```python
from build123d import *

# Parameters (mm, degrees)
SKETCH1_R           = 3.75
SKETCH1_R_2         = 1.6
BOSS_EXTRUDE1_DEPTH = 2
BOSS_EXTRUDE2_START = -15
BOSS_EXTRUDE2_DEPTH = 15
BOSS_EXTRUDE3_DEPTH = 2
SKETCH2_R           = 2
CUT_EXTRUDE1_DEPTH  = 39.169212171
CUT_EXTRUDE2_START  = -4
SKETCH2_3_R         = 2
CUT_EXTRUDE2_DEPTH  = 35.169212171


# Read off the part's stored shape, not the designer's step: Boss-Extrude2
with BuildPart() as part:
    # Sketch1 → Boss-Extrude1 (new body)
    # profile 1 of 5: a face of its own
    with BuildSketch(Plane.XY):
        with Locations((-33.25, 6.273123532)):
            Circle(SKETCH1_R)
        with Locations((-33.25, 6.273123532)):
            Circle(SKETCH1_R_2, mode=Mode.SUBTRACT)
    # profile 2 of 5: a face of its own
    with BuildSketch(Plane.XY):
        with BuildLine():
            Line((0, 2.523123532), (3.75, 2.523123532))
            ThreePointArc((3.75, 2.523123532), (0.004577287, 6.087897443), (3.38, 10.004825556))
            Line((3.38, 10.004825556), (0, 10.023123532))
            Line((0, 10.023123532), (0, 13))
            Line((0, 13), (-29.5, 13))
            Line((-29.5, 13), (-29.5, 10.023123532))
            Line((-29.5, 10.023123532), (-33.25, 10.023123532))
            ThreePointArc((-33.25, 10.023123532), (-30.598349571, 8.924773961), (-29.5, 6.273123532))
            ThreePointArc((-29.5, 6.273123532), (-30.598349571, 3.621473102), (-33.25, 2.523123532))
            Line((-33.25, 2.523123532), (-29.5, 2.523123532))
            Line((-29.5, 2.523123532), (-29.5, 0))
            Line((-29.5, 0), (0, 0))
            Line((0, 0), (0, 2.523123532))
        make_face()
    # profile 3 of 5: a face of its own
    with BuildSketch(Plane.XY):
        with Locations((3.75, 6.273123532)):
            Circle(SKETCH1_R)
        with Locations((3.75, 6.273123532)):
            Circle(SKETCH1_R_2, mode=Mode.SUBTRACT)
    # profile 4 of 5: a face of its own
    with BuildSketch(Plane.XY):
        with BuildLine():
            ThreePointArc((7.5, 6.273123532), (6.401650429, 3.621473102), (3.75, 2.523123532))
            Line((3.75, 2.523123532), (0, 2.523123532))
            Line((0, 2.523123532), (0, 0))
            Line((0, 0), (7.5, 0))
            Line((7.5, 0), (7.5, 6.273123532))
        make_face()
    # profile 5 of 5: a face of its own
    with BuildSketch(Plane.XY):
        with BuildLine():
            Line((-37, 0), (-29.5, 0))
            Line((-29.5, 0), (-29.5, 2.523123532))
            Line((-29.5, 2.523123532), (-33.25, 2.523123532))
            ThreePointArc((-33.25, 2.523123532), (-35.901650429, 3.621473102), (-37, 6.273123532))
            Line((-37, 6.273123532), (-37, 0))
        make_face()
    extrude(amount=BOSS_EXTRUDE1_DEPTH)



with BuildPart() as body_2:
    # Boss-Extrude2 outline → Boss-Extrude2 (new body)
    with BuildSketch(Plane(origin=(0, 0, 0), x_dir=(1, 0, 0), z_dir=(0, 1, 0)).offset(BOSS_EXTRUDE2_START)):
        Polygon((7.5, 0), (7.5, 26.552667029), (-37, 5.801976241), (-37, 0), align=None)
    extrude(amount=BOSS_EXTRUDE2_DEPTH)


with BuildPart() as part_1:
    add(part.part)

    add(body_2.part)  # Boss-Extrude3 merges body 2
    # Sketch1<5> → Boss-Extrude3 (add)
    with BuildSketch(Plane.XY):
        Polygon((7.5, 0), (0, 0), (-29.5, 0), (-37, 0), (-37, -15), (7.5, -15), align=None)
    extrude(amount=BOSS_EXTRUDE3_DEPTH)

    # Sketch2 → Cut-Extrude1 (cut, through all)
    with BuildSketch(Plane(origin=(-8.83071505, 0, -18.937529538), x_dir=(-0.9063077870366508, 0, 0.42261826174069766), z_dir=(-0.4226182617406977, 1.198406961524809e-15, -0.9063077870366509))):
        with Locations((16.531049613, -7.5)):
            Circle(SKETCH2_R)
        with Locations((-3.468950387, -7.5)):
            Circle(SKETCH2_R)
    extrude(amount=-CUT_EXTRUDE1_DEPTH, mode=Mode.SUBTRACT)

    # Sketch2<3> → Cut-Extrude2 (cut, through all)
    # profile 1 of 2: a face of its own
    with BuildSketch(Plane(origin=(-8.83071505, 0, -18.937529538), x_dir=(-0.9063077870366508, 0, 0.42261826174069766), z_dir=(-0.4226182617406977, 1.198406961524809e-15, -0.9063077870366509)).offset(CUT_EXTRUDE2_START)):
        Polygon((12.605067782, -7.5), (14.568058697, -10.9), (18.494040528, -10.9), (20.457031443, -7.5), (18.494040528, -4.1), (14.568058697, -4.1), align=None)
        with Locations((16.531049613, -7.5)):
            Circle(SKETCH2_3_R, mode=Mode.SUBTRACT)
    # profile 2 of 2: a face of its own
    with BuildSketch(Plane(origin=(-8.83071505, 0, -18.937529538), x_dir=(-0.9063077870366508, 0, 0.42261826174069766), z_dir=(-0.4226182617406977, 1.198406961524809e-15, -0.9063077870366509)).offset(CUT_EXTRUDE2_START)):
        Polygon((-5.431941303, -4.1), (-7.394932218, -7.5), (-5.431941303, -10.9), (-1.505959472, -10.9), (0.457031443, -7.5), (-1.505959472, -4.1), align=None)
        with Locations((-3.468950387, -7.5)):
            Circle(SKETCH2_3_R, mode=Mode.SUBTRACT)
    extrude(amount=-CUT_EXTRUDE2_DEPTH, mode=Mode.SUBTRACT)


solid = part_1.part
```
Geometry: final body of the model. Coordinates: model frame, mm. A direction names the side the tool comes from. Round coordinates to 2 decimals unless told otherwise and drop trailing zeros. Order: outer loops, then holes, each group sorted by start corner. A loop starts at its lowest first (then second) coordinate and runs counter-clockwise, first axis right, second up. Notation, with made-up numbers: M 44,36 L 92,36 A37 ccw 92,73 Z; hole C 32,21.5 d1. An arc over 180 degrees is marked long. Use one line per item in the form item = value. Start each with the question number.
Q1. Cut plane B-B (x = -14.5). Return loops of the section in (y, z), and give its area (3 significant figures).
Q2. Cut plane C-C (z = -5). Return loops of the section in (x, y), and give its area (3 significant figures).
Q3. Cut plane D-D (y = -0.5). Return loops of the section in (x, z), and give its area (3 significant figures).
Q4. Cut plane A-A (y = -8.5). Return loops of the section in (x, z), and give its area (3 significant figures).
Q5. Mould query, pull axis Y, two halves, no side actions, for faces 6 (the face through (-15, 13, 1)), 7 (the face through (-20, -10.9, -3)), 8 (the face through (-29.5, 12, 1)). Classes: +Y half, -Y half, draft (parallel to the pull), parting line (faces both ways), or undercut.
Q6. Material intervals for line 1 (Y direction, x = 3.75, z = 1.5); line 2 (Y direction, x = -33.25, z = 1.4); line 3 (Z direction, x = -12.5, y = 10.75), sorted ascending. Write a range as [from, to].
Q7. Pin query (flat end, axial travel): pin 1 Ø4 at (x, y) = (-33.25, 6.27) entering from -Z; pin 2 Ø4 at (x, z) = (-0.5, -5.5) entering from +Y; pin 3 Ø1 at (x, z) = (-30.5, 1) entering from +Y. Return the tip coordinate at first contact, or that it passes through.
Q8. Access query for faces 1 (the face through (-5.528, -5.941, -16.064)), 2 (the face through (-15, 7, 0)), 3 (the face through (-34.85, 6.34, 0.99)), 4 (the face through (-31, 10.023, 1)), 5 (the face through (-15, -1, 2)). Directions: +Z, -Z, +X, -X, +Y, -Y. A direction counts if a zero-diameter tool reaches every point of the face in a straight line with its end or side. Return the directions, or none.
Geometry results:
q1.outline = M -15,-16.29 L 0,-16.29 L 0,0 L 13,0 L 13,2 L -5.11,2 L -7.5,-1.27 L -9.89,2 L -15,2 Z
q1.area = 293 mm^2
q2.outline = M -37,-15 L 7.5,-15 L 7.5,0 L -37,0 Z; hole M -24.9,-7.5 L -22.74,-10.9 L -18.41,-10.9 L -16.24,-7.5 L -18.41,-4.1 L -22.74,-4.1 Z; hole M -2.84,-7.5 L -0.67,-10.9 L 3.66,-10.9 L 5.83,-7.5 L 3.66,-4.1 L -0.67,-4.1 Z
q2.area = 579 mm^2
q3.outline = M -37,-5.8 L 7.5,-26.55 L 7.5,2 L -37,2 Z
q3.area = 809 mm^2
q4.outline = M -37,-5.8 L -25.38,-11.22 L -23.69,-7.59 L -25.16,-6.91 L -21,2 L -37,2 Z; M -22.24,-12.68 L -7.26,-19.67 L -5.57,-16.05 L -7.03,-15.36 L 1.07,2 L -13.61,2 L -19.09,-9.74 L -20.55,-9.06 Z; M -4.12,-21.14 L 7.5,-26.55 L 7.5,-0.05 L -0.96,-18.19 L -2.43,-17.51 Z
q4.area = 567 mm^2
q5.face_6 = +Y half
q5.face_7 = undercut
q5.face_8 = draft
q6.line_1 = [-15, -10.9], [-4.1, 4.67], [7.87, 10.02]
q6.line_2 = [-15, 4.67], [7.87, 10.02]
q6.line_3 = [0, 2]
q7.pin_1 = 0
q7.pin_2 = 0
q7.pin_3 = 10.02
q8.face_1 = none
q8.face_2 = -Z, +X, -X, +Y
q8.face_3 = +Z, -Z
q8.face_4 = +Z, -Z, -X, +Y
q8.face_5 = +Z, +X, -X, +Y, -Y
